```python
from build123d import *

# Parameters (mm, degrees)
SKETCH_1_W      = 13
SKETCH_1_H      = 13
SKETCH_1_R      = 4.95
EXTRUDE_1_DEPTH = 1
SKETCH_2_W      = 13
SKETCH_2_H      = 13
SKETCH_2_W_2    = 9.2
SKETCH_2_H_2    = 9.2
EXTRUDE_2_DEPTH = 2.5
SKETCH_3_W      = 8.5
SKETCH_3_H      = 6
SKETCH_3_R      = 1.6
EXTRUDE_3_DEPTH = 3.5


with BuildPart() as part:
    # 草图1 → 凸台-拉伸1 (new body)
    with BuildSketch(Plane.XY):
        with Locations((-0.565783989, 1.095956893)):
            Rectangle(SKETCH_1_W, SKETCH_1_H)
        with Locations((-0.565783989, 1.095956893)):
            Circle(SKETCH_1_R, mode=Mode.SUBTRACT)
    extrude(amount=EXTRUDE_1_DEPTH)

    # 草图2 → 凸台-拉伸2 (add)
    with BuildSketch(Plane.XY.offset(1)):
        with Locations((-0.565783989, 1.095956893)):
            Rectangle(SKETCH_2_W, SKETCH_2_H)
        with Locations((-0.565783989, 1.095956893)):
            Rectangle(SKETCH_2_W_2, SKETCH_2_H_2, mode=Mode.SUBTRACT)
    extrude(amount=EXTRUDE_2_DEPTH)

    # 草图3 → 凸台-拉伸3 (add)
    with BuildSketch(Plane.XY.offset(3.5)):
        with Locations((10.184216011, 2.695956893)):
            Rectangle(SKETCH_3_W, SKETCH_3_H)
        with Locations((10.934216011, 2.195956893)):
            Circle(SKETCH_3_R, mode=Mode.SUBTRACT)
        with Locations((-11.315783989, 2.695956893)):
            Rectangle(SKETCH_3_W, SKETCH_3_H)
        with Locations((-12.065783989, 2.195956893)):
            Circle(SKETCH_3_R, mode=Mode.SUBTRACT)
    extrude(amount=-EXTRUDE_3_DEPTH)


solid = part.part
```
Can you work these out from the model? Positions are in its coordinate system, mm. A direction names the side the tool comes from. Give positions to 0.01 mm unless a question says otherwise; leave off trailing zeros. Loops run counter-clockwise (first coordinate to the right, second up) from the corner with the lowest first, then second, coordinate; pieces in that order, holes last. Notation, with made-up numbers: M 81,40.25 L 122,40.25 A15 cw 122,56.25 Z; hole C 4.5,31 d7. An arc over 180 degrees is marked long. Answer in a Markdown table with one row per item.
1. Thinking about a two-plate mould opening in X: for faces 4 (the flat face through (-1, -3.504, 2)), 5 (the flat face through (-11, 5.696, 2)), 6 (the flat face through (5.934, 7, 2)), which applies, released by +X, released by -X, zero draft, split by the parting line, or undercut?
Taken from the geometry:
| item | result |
|---|---|
| face 4 | undercut |
| face 5 | zero draft |
| face 6 | released by +X |
2. Which directions (+Z, -Z, +X, -X, +Y, -Y) give clear straight access to the entire face, cutting with the end or side of a thin tool? Please do faces 1 (the flat face through (10, 5.696, 2)), 2 (the flat face through (-11, -0.304, 2)), 3 (the flat face through (-5.166, 1, 2)).
Taken from the geometry:
| item | result |
|---|---|
| face 1 | +Z, -Z, +X, +Y |
| face 2 | +Z, -Z, -X, -Y |
| face 3 | +Z |
3. Suppose I cut it at C-C on z = 1.3. Write out the boundary of the cut face in (x, y), plus the area to 3 significant figures.
Taken from the geometry:
| item | result |
|---|---|
| outline | M -15.57,-0.3 L -7.07,-0.3 L -7.07,-5.4 L 5.93,-5.4 L 5.93,-0.3 L 14.43,-0.3 L 14.43,5.7 L 5.93,5.7 L 5.93,7.6 L -7.07,7.6 L -7.07,5.7 L -15.57,5.7 Z; hole C -12.07,2.2 d3.2; hole M -5.17,-3.5 L 4.03,-3.5 L 4.03,5.7 L -5.17,5.7 Z; hole C 10.93,2.2 d3.2 |
| area | 170 mm² |
4. Suppose I cut it at B-B on x = 2.25. Write out the boundary of the cut face in (y, z), plus the area to 3 significant figures.
Taken from the geometry:
| item | result |
|---|---|
| outline | M -5.4,0 L -2.98,0 L -2.98,1 L -3.5,1 L -3.5,3.5 L -5.4,3.5 Z; M 5.17,0 L 7.6,0 L 7.6,3.5 L 5.7,3.5 L 5.7,1 L 5.17,1 Z |
| area | 14.4 mm² |
5. If I drill on line 1 along Y through (x, z) = (0.25, 1.75); line 2 along X through (y, z) = (-3, 1.7); line 3 along X through (y, z) = (2, 1.25), over which ranges is the centre line in solid material (lowest first)?
Taken from the geometry:
| item | result |
|---|---|
| line 1 | y = -5.4 to -3.5, 5.7 to 7.6 |
| line 2 | x = -7.07 to -5.17, 4.03 to 5.93 |
| line 3 | x = -15.57 to -13.65, -10.48 to -5.17, 4.03 to 9.35, 12.52 to 14.43 |
6. Suppose I cut it at A-A on y = 0.25. Write out the boundary of the cut face in (x, z), plus the area to 3 significant figures.
Taken from the geometry:
| item | result |
|---|---|
| outline | M -15.57,0 L -5.44,0 L -5.44,1 L -5.17,1 L -5.17,3.5 L -15.57,3.5 Z; M 4.03,1 L 4.31,1 L 4.31,0 L 14.43,0 L 14.43,3.5 L 4.03,3.5 Z |
| area | 72.2 mm² |
7. For pin 1 Ø1 at (y, z) = (6.5, 2) entering from -X; pin 2 Ø1.8 at (x, z) = (-11.5, 1.5) entering from +Y; pin 3 Ø1.5 at (x, z) = (-8.5, 2.5) entering from -Y, each with a flat end and sliding along its axis, tell me the tip position at first contact or that it passes through.
Taken from the geometry:
| item | result |
|---|---|
| pin 1 | stops at x = -7.07 |
| pin 2 | stops at y = 5.7 |
| pin 3 | stops at y = -0.3 |
8. Suppose I cut it at D-D on x = -9. Write out the boundary of the cut face in (y, z), plus the area to 3 significant figures.
Taken from the geometry:
| item | result |
|---|---|
| outline | M -0.3,0 L 5.7,0 L 5.7,3.5 L -0.3,3.5 Z |
| area | 21.0 mm² |
